Design review of the part built by this model. Coordinates are the model's own, in mm. Give positions to 0.01 mm unless a question says otherwise; leave off trailing zeros. Write each loop counter-clockwise with the first axis right and the second up, starting at its lowest first coordinate (ties: lowest second). Pieces come first, ordered by that corner, then holes. Notation, with made-up numbers: M 74,72.5 L 97,72.5 A4 cw 97,76.5 Z; hole C 2.5,89 d2. An arc over 180 degrees is marked long. Answer in a Markdown table with one row per item.
Autodesk Inventor part; units mm, degrees
ref_plane "YZ Plane" through (0, 0, 0) normal (1, 0, 0) x (0, 1, 0)
ref_plane "XZ Plane" through (0, 0, 0) normal (0, 1, 0) x (-1, 0, 0)
ref_plane "XY Plane" through (0, 0, 0) normal (0, 0, 1) x (1, 0, 0)
sketch "Sketch1" plane through (0, 0, 0) normal (0, 1, 0) x (-1, 0, 0)
  point P0 (0, 0)
sketch "Sketch2" plane through (0, 0, 0) normal (0, 1, 0) x (-1, 0, 0)
  circle A0 centre (0, 0) radius 8
  circle A1 centre (0, 0) radius 15
  dimension "d0" = 16
  dimension "d1" = 30
extrude "Extrusion1" add sketch "Sketch2" along normal blind 15
fillet "Fillet1" radius 2 1 edges at (15, 15, 0)
fillet "Fillet2" radius 2 1 edges at (8, 15, 0)
fillet "Fillet3" radius 2 2 edges at (15, 0, 0) (8, 0, 0)
properties part number "coil"
1) The part is to be moulded in two halves that separate along Z. For faces 1 (the face through (14.985, 7.423, -0.66)), 2 (the face through (1.73, 7.42, 7.81)), 3 (the face through (-7, 0, -8)), say which applies: released by +Z, released by -Z, zero draft, split by the parting line, or undercut.
Geometry says:
| item | result |
|---|---|
| face 1 | split by the parting line |
| face 2 | undercut |
| face 3 | zero draft |
2) Add section B-B (z = 0). Write out the cut boundary in (x, y).
Geometry says:
| item | result |
|---|---|
| outline | M -15,2 A2 ccw -13,0 L -10,0 A2 ccw -8,2 L -8,13 A2 ccw -10,15 L -13,15 A2 ccw -15,13 Z; M 8,2 A2 ccw 10,0 L 13,0 A2 ccw 15,2 L 15,13 A2 ccw 13,15 L 10,15 A2 ccw 8,13 Z |
3) Add section A-A (x = 0). Write out the cut boundary in (y, z), and give its area (3 significant figures).
Geometry says:
| item | result |
|---|---|
| outline | M 0,-13 A2 ccw 2,-15 L 13,-15 A2 ccw 15,-13 L 15,-10 A2 ccw 13,-8 L 2,-8 A2 ccw 0,-10 Z; M 0,10 A2 ccw 2,8 L 13,8 A2 ccw 15,10 L 15,13 A2 ccw 13,15 L 2,15 A2 ccw 0,13 Z |
| area | 203 mm^2 |
4) Insertion check: P1, Ø1.5, axis at x = 3, z = 5, coming from the -Y side; P2, Ø1, axis at x = 5, y = 13.5, coming from the -Z side; P3, Ø1, axis at y = 3, z = -9, coming from the +X side; P4, Ø3, axis at x = -8.5, y = 9.5, coming from the -Z side. Each pin has a flat end and moves straight along its axis. Give the tip position at first contact, or say it passes through.
Geometry says:
| item | result |
|---|---|
| P1 | through |
| P2 | z = -14.27 |
| P3 | x = 12.36 |
| P4 | z = -13.27 |
5) To check wall thickness, follow probe 1 along Z at (x, y) = (0, 8.5); probe 2 along Y at (x, z) = (-6, 7.75); probe 3 along Z at (x, y) = (-6.25, 9.25). State the ranges of each line that lie inside material, in increasing order. Write a range as [from, to].
Geometry says:
| item | result |
|---|---|
| probe 1 | [-15, -8], [8, 15] |
| probe 2 | [0.01, 14.99] |
| probe 3 | [-13.64, -4.99], [4.99, 13.64] |
6) Add section C-C (y = 5.25). Write out the cut boundary in (x, z), and give its area (3 significant figures).
Geometry says:
| item | result |
|---|---|
| outline | C 0,0 d30; hole C 0,0 d16 |
| area | 506 mm^2 |
